Autodesk Inventor part; units mm, degrees
ref_plane "YZ Plane" through (0, 0, 0) normal (1, 0, 0) x (0, 1, 0)
ref_plane "XZ Plane" through (0, 0, 0) normal (0, 1, 0) x (-1, 0, 0)
ref_plane "XY Plane" through (0, 0, 0) normal (0, 0, 1) x (1, 0, 0)
sketch "Sketch1" plane through (0, 0, 0) normal (0, 1, 0) x (-1, 0, 0)
  circle A0 centre (0, 0) radius 30
  circle A1 centre (0, 0) radius 20
  dimension "d0" = 60
  dimension "d1" = 40
extrude "Extrusion1" add sketch "Sketch1" along normal blind 60
sketch "Sketch2" plane through (0, 0, 0) normal (0, -1, 0) x (1, 0, 0)
  circle A0 centre (75, 0) radius 10
  arc A1 (75, -23) -> (75, 23) centre (75, 0) ccw
  circle A2 centre (0, 0) radius 30
  line L0 (19.2614, 23) -> (75, 23)
  line L1 (19.2614, -23) -> (75, -23)
  dimension "d4" = 20
  dimension "d5" = 46
  dimension "d8" = 75
extrude "Extrusion2" add sketch "Sketch2" against normal blind 15 contours L1 A2 L0 A1
sketch "Sketch3" plane through (0, 15, 0) normal (0, 1, 0) x (1, 0, 0)
  line L0 (-75, -30) -> (0, -30)
  line L1 (0, -30) -> (0, 30)
  line L2 (0, 30) -> (-75, 30)
  line L3 (-75, 30) -> (-75, -30)
  arc A0 (19.2614, 23) -> (19.2614, -23) centre (0, 0) ccw
  dimension "d11" = 60
  dimension "d12" = 75
extrude "Extrusion3" add sketch "Sketch3" along normal blind 15 contours L3 L2 A0 L0
sketch "Sketch4" plane through (0, 30, 0) normal (0, 1, 0) x (1, 0, 0)
  line L0 (-75, 30) -> (-60, 30)
  line L1 (-60, 30) -> (-60, -30)
  line L2 (-60, -30) -> (-75, -30)
  line L3 (-75, -30) -> (-75, 30)
  line L4 (0, 30) -> (-75, 30)
  line L5 (-75, 30) -> (-75, -30)
  line L6 (-75, -30) -> (0, -30)
  line L7 (-60, 5) -> (-29.5804, 5)
  line L8 (-29.5804, 5) -> (-29.5804, -5)
  line L9 (-29.5804, -5) -> (-60, -5)
  line L10 (-60, -5) -> (-60, 5)
  circle A0 centre (0, 0) radius 30
  dimension "d15" = 15
  dimension "d16" = 10
extrude "Extrusion4" add sketch "Sketch4" along normal blind 30 contours L0 L1 L2 L3 | L7 A0 L9 L1 | L8 A0 picked at (-29.7047, 0.5579)
sketch "Sketch5" plane through (-75, 15, -30) normal (-1, 0, 0) x (0, 0, 1)
  circle A0 centre (12.5, 30) radius 8
  circle A1 centre (47.5, 30) radius 8
  line L0 (60, 0) -> (60, 45)
  line L1 (0, 45) -> (60, 45)
  point P0 (30, -15)
  dimension "d19" = 16
  dimension "d20" = 35
  dimension "d21" = 12.5
  dimension "d22" = 15
extrude "Extrusion5" cut sketch "Sketch5" against normal up to surface (15 mm away)
sketch "Sketch6" plane through (0, 0, 0) normal (0, 0, 1) x (1, 0, 0)
  line L0 (29.615, 55) -> (29.615, 15)
  line L1 (29.615, 15) -> (54.615, 15)
  line L2 (54.615, 15) -> (29.615, 55)
  line L3 (19.2614, 15) -> (75, 15)
  line L4 (29.998, 59.9996) -> (29.998, 15) construction
  point P0 (0, 0)
  dimension "d25" = 25
  dimension "d26" = 40
  dimension "d27" = 0.383
extrude "Extrusion6" add sketch "Sketch6" along normal mid plane 10
properties part number "Exercise03"
Part model, mm, in its own coordinate system. A direction names the side the tool comes from. Give positions to 0.01 mm unless a question says otherwise; leave off trailing zeros. Loops run counter-clockwise (first coordinate to the right, second up) from the corner with the lowest first, then second, coordinate; pieces in that order, holes last. Notation, with made-up numbers: M 39.5,-5 L 62.5,-5 A7 ccw 62.5,3 Z; hole C -24,38.5 d5. An arc over 180 degrees is marked long. Put each result on its own line as item: value. Start each with the question number.
1) Saw through at D-D (y = 26). List the corners of the cut face in (x, z) (3 decimals).
2) Probe probe 1 along X at (y, z) = (56.5, 16); probe 2 along X at (y, z) = (43, 5.5); probe 3 along Z at (x, y) = (0, 13.5). List the from-to ranges inside material, lowest first.
3) 3-axis set-ups, long thin cutter, end or side, ignore diameter. For faces 4 (the flat face through (47, 7, 23)), 5 (the cylindrical face through (-67.605, 52.932, -18.541)), 6 (the flat face through (47, 7, -23)), 7 (the flat face through (36, 26, -5)), 8 (the flat face through (36, 26, 5)): which of +Z, -Z, +X, -X, +Y, -Y reach the whole face in a straight line?
4) Saw through at C-C (z = 0). List the corners of the cut face in (x, y) (3 decimals).
5) Saw through at B-B (x = -62). List the corners of the cut face in (y, z), then the cut area to 3 significant figures.
6) Saw through at A-A (y = 41.5). State how many separate pieces and enclosed holes the cut face has, then the cut area to 3 significant figures.
7) Flat gauge pins, fed straight in: pin 1 (1.5 mm diameter, centred on x = 36, y = 36.5, fed in from -Z); pin 2 (7.5 mm diameter, centred on x = 35.5, y = 9, fed in from +Z); pin 3 (12.5 mm diameter, centred on x = -35, z = -17, fed in from +Y). Where does each tip first touch, or does it go through?
8) Pull direction X, two halves, no side cores. Call faces 1 (the flat face through (42.29, 34.72, -0.07)), 2 (the flat face through (-45, 27, -30)), 3 (the flat face through (-44, 30, 17)): +X half, -X half, draft (parallel to the pull), parting line (faces both ways), or undercut.
Numbers:
1. outline: M -75,-30 L 0,-30 A30 ccw 29.615,-4.791 L 29.615,-5 L 47.74,-5 L 47.74,5 L 29.615,5 L 29.615,4.791 A30 ccw 0,30 L -75,30 Z; hole C 0,0 d40
2. probe 1: -75 to -60, -25.38 to -12, 12 to 25.38
2. probe 2: -75 to -60, -29.49 to -19.23, 19.23 to 29.49
2. probe 3: -30 to -20, 20 to 30
3. face 4: +Z, +X, +Y, -Y
3. face 5: -X
3. face 6: -Z, +X, +Y, -Y
3. face 7: -Z, +X, +Y
3. face 8: +Z, +X, +Y
4. outline: M -75,15 L -30,15 L -30,0 L -20,0 L -20,60 L -75,60 Z; M 20,0 L 65,0 L 65,15 L 54.615,15 L 30,54.384 L 30,60 L 20,60 Z; M 85,0 L 98,0 L 98,15 L 85,15 Z
5. outline: M 15,-30 L 60,-30 L 60,30 L 15,30 Z; hole C 45,-17.5 d16; hole C 45,17.5 d16
5. area: 2,300 mm^2
6. separate pieces: 3
6. enclosed holes: 1
6. area: 2,420 mm^2
7. pin 1: z = -5
7. pin 2: z = 23
7. pin 3: y = 30
8. face 1: +X half
8. face 2: draft
8. face 3: undercut
